from build123d import *

# Parameters (mm, degrees)
MAIN_PLATE_DEPTH                         = 1
LONG_EDGE_DEPTH                          = 251
LONG_EDGE_FILLETS_R                      = 10
M4_CLEARANCE_HOLE1_D                     = 4.5
M4_CLEARANCE_HOLE1_DEPTH                 = 178
SHORT_EDGE_DEPTH                         = 171
SHORT_EDGE_FILLETS_R                     = 10
M4_CLEARANCE_HOLE2_D                     = 4.5
M4_CLEARANCE_HOLE2_DEPTH                 = 258
LONG_EDGE_FILLETS_OF_OTHER_LONG_EDGE_R   = 10
SHORT_EDGE_FILLETS_OF_OTHER_SHORT_EDGE_R = 10


# Sheet-metal steps are written as plain solids
with BuildPart() as part:
    # Sketch1 → Main Plate (new body)
    with BuildSketch(Plane.XY):
        Polygon((-126.5, -85.5), (-125.5, -86.5), (125.5, -86.5), (126.5, -85.5), (126.5, 85.5), (125.5, 86.5), (-125.5, 86.5), (-126.5, 85.5), align=None)
    extrude(amount=-MAIN_PLATE_DEPTH)

    # Long Edge section (across the edge) → Long Edge (add)
    with BuildSketch(Plane(origin=(-125.5, 88, -1), x_dir=(0, -1, 0), z_dir=(1, 0, 0))):
        with BuildLine():
            Line((-1, 1.5), (-1, 17))
            Line((-1, 17), (0, 17))
            Line((0, 17), (0, 1.5))
            ThreePointArc((0, 1.5), (0.439339828, 0.439339828), (1.5, 0))
            Line((1.5, 0), (1.5, -1))
            ThreePointArc((1.5, -1), (-0.267766953, -0.267766953), (-1, 1.5))
        make_face()
    long_edge = extrude(amount=LONG_EDGE_DEPTH)

    # Long Edge Fillets
    long_edge_fillets_edges = [part.edges().sort_by_distance(p)[0] for p in [
        (-125.5, 88.5, -18),
        (125.5, 88.5, -18),
    ]]
    fillet(long_edge_fillets_edges, radius=LONG_EDGE_FILLETS_R)

    # M4 Clearance Hole1
    with Locations(Plane(origin=(0, 89, 0), x_dir=(1, 0, 0), z_dir=(0, 1, 0))):
        with Locations((-115.5, 10), (115.5, 10), (0, 10)):
            m4_clearance_hole1 = Hole(M4_CLEARANCE_HOLE1_D / 2, depth=M4_CLEARANCE_HOLE1_DEPTH)

    # Short Edge section (across the edge) → Short Edge (add)
    with BuildSketch(Plane(origin=(128, 85.5, -1), x_dir=(-1, 0, 0), z_dir=(0, -1, 0))):
        with BuildLine():
            Line((-1, 1.5), (-1, 17))
            Line((-1, 17), (0, 17))
            Line((0, 17), (0, 1.5))
            ThreePointArc((0, 1.5), (0.439339828, 0.439339828), (1.5, 0))
            Line((1.5, 0), (1.5, -1))
            ThreePointArc((1.5, -1), (-0.267766953, -0.267766953), (-1, 1.5))
        make_face()
    short_edge = extrude(amount=SHORT_EDGE_DEPTH)

    # Short Edge Fillets
    short_edge_fillets_edges = [part.edges().sort_by_distance(p)[0] for p in [
        (128.5, 85.5, -18),
        (128.5, -85.5, -18),
    ]]
    fillet(short_edge_fillets_edges, radius=SHORT_EDGE_FILLETS_R)

    # M4 Clearance Hole2
    with Locations(Plane(origin=(129, 0, 0), x_dir=(0, 0, -1), z_dir=(1, 0, 0))):
        with Locations((10, -75.5), (10, 75.5)):
            m4_clearance_hole2 = Hole(M4_CLEARANCE_HOLE2_D / 2, depth=M4_CLEARANCE_HOLE2_DEPTH)

    # Other Long Edge: Long Edge, M4 Clearance Hole1 across plane
    add(long_edge.mirror(Plane.ZX))
    add(m4_clearance_hole1.mirror(Plane.ZX), mode=Mode.SUBTRACT)

    # Long Edge Fillets of Other Long Edge
    long_edge_fillets_of_other_long_edge_edges = [part.edges().sort_by_distance(p)[0] for p in [
        (-125.5, -88.5, -18),
        (125.5, -88.5, -18),
    ]]
    fillet(long_edge_fillets_of_other_long_edge_edges, radius=LONG_EDGE_FILLETS_OF_OTHER_LONG_EDGE_R)

    # Other Short Edge: Short Edge, M4 Clearance Hole2 across plane
    add(short_edge.mirror(Plane(origin=(0, 0, 0), x_dir=(0, 0, 1), z_dir=(1, 0, 0))))
    add(m4_clearance_hole2.mirror(Plane(origin=(0, 0, 0), x_dir=(0, 0, 1), z_dir=(1, 0, 0))), mode=Mode.SUBTRACT)

    # Short Edge Fillets of Other Short Edge
    short_edge_fillets_of_other_short_edge_edges = [part.edges().sort_by_distance(p)[0] for p in [
        (-128.5, 85.5, -18),
        (-128.5, -85.5, -18),
    ]]
    fillet(short_edge_fillets_of_other_short_edge_edges, radius=SHORT_EDGE_FILLETS_OF_OTHER_SHORT_EDGE_R)


solid = part.part
Can you work these out from the model? Positions are in its coordinate system, mm. A direction names the side the tool comes from. Round coordinates to 2 decimals unless told otherwise and drop trailing zeros. Order: outer loops, then holes, each group sorted by start corner. A loop starts at its lowest first (then second) coordinate and runs counter-clockwise, first axis right, second up. Notation, with made-up numbers: M 50.5,-13 L 75.5,-13 A6 cw 75.5,-4 Z; hole C 86,8.25 d4. An arc over 180 degrees is marked long. Use a Markdown table: item, result.
1) I'm going to push flat-ended pins straight in: P1, Ø1.2, axis at y = 88, z = -2.5, coming from the +X side; P2, Ø2, axis at x = 128, z = -5, coming from the +Y side; P3, Ø3, axis at x = -128.5, z = -3, coming from the -Y side. Where does each tip first touch, or does it pass through?
Geometry says:
| item | result |
|---|---|
| P1 | stops at x = 125.5 |
| P2 | stops at y = 85.5 |
| P3 | stops at y = -85.5 |
2) Imagine slicing it at B-B (x = 56.5). List the corners of the cut face in (y, z) for me, then the cut area to 3 significant figures.
Geometry says:
| item | result |
|---|---|
| outline | M -89,-18 L -88,-18 L -88,-2.5 A1.5 cw -86.5,-1 L 86.5,-1 A1.5 cw 88,-2.5 L 88,-18 L 89,-18 L 89,-2.5 A2.5 ccw 86.5,0 L -86.5,0 A2.5 ccw -89,-2.5 Z |
| area | 210 mm² |
3) Imagine slicing it at A-A (y = -9). List the corners of the cut face in (x, z) for me.
Geometry says:
| item | result |
|---|---|
| outline | M -129,-18 L -128,-18 L -128,-2.5 A1.5 cw -126.5,-1 L 126.5,-1 A1.5 cw 128,-2.5 L 128,-18 L 129,-18 L 129,-2.5 A2.5 ccw 126.5,0 L -126.5,0 A2.5 ccw -129,-2.5 Z |
4) If I drill on line 1 along Y through (x, z) = (-38.5, -11.25); line 2 along X through (y, z) = (-11.5, -7.5); line 3 along X through (y, z) = (88.2, -10), over which ranges is the centre line in solid material (lowest first)?
Geometry says:
| item | result |
|---|---|
| line 1 | y = -89 to -88, 88 to 89 |
| line 2 | x = -129 to -128, 128 to 129 |
| line 3 | x = -125.3 to -117.75, -113.25 to -2.25, 2.25 to 113.25, 117.75 to 125.3 |
5) On a 3-axis mill with a long thin cutter (end or side, diameter ignored), from which of +Z, -Z, +X, -X, +Y, -Y can I reach the whole of each face in a straight line? I mean faces 1 (the face through (128, 1, -10)), 2 (the face through (-2, -88, -12)), 3 (the face through (-2, 1, -1)). Say none if no direction works.
Geometry says:
| item | result |
|---|---|
| face 1 | -Z, +Y, -Y |
| face 2 | -Z, +X, -X |
| face 3 | -Z |
